Geometry check sheet. Reference: drawing and pictorial views, mm from the part's lowest x, y, z. A direction names the side the tool comes from. Give positions to 0.01 mm unless a question says otherwise; leave off trailing zeros. Write each loop counter-clockwise with the first axis right and the second up, starting at its lowest first coordinate (ties: lowest second). Pieces come first, ordered by that corner, then holes.
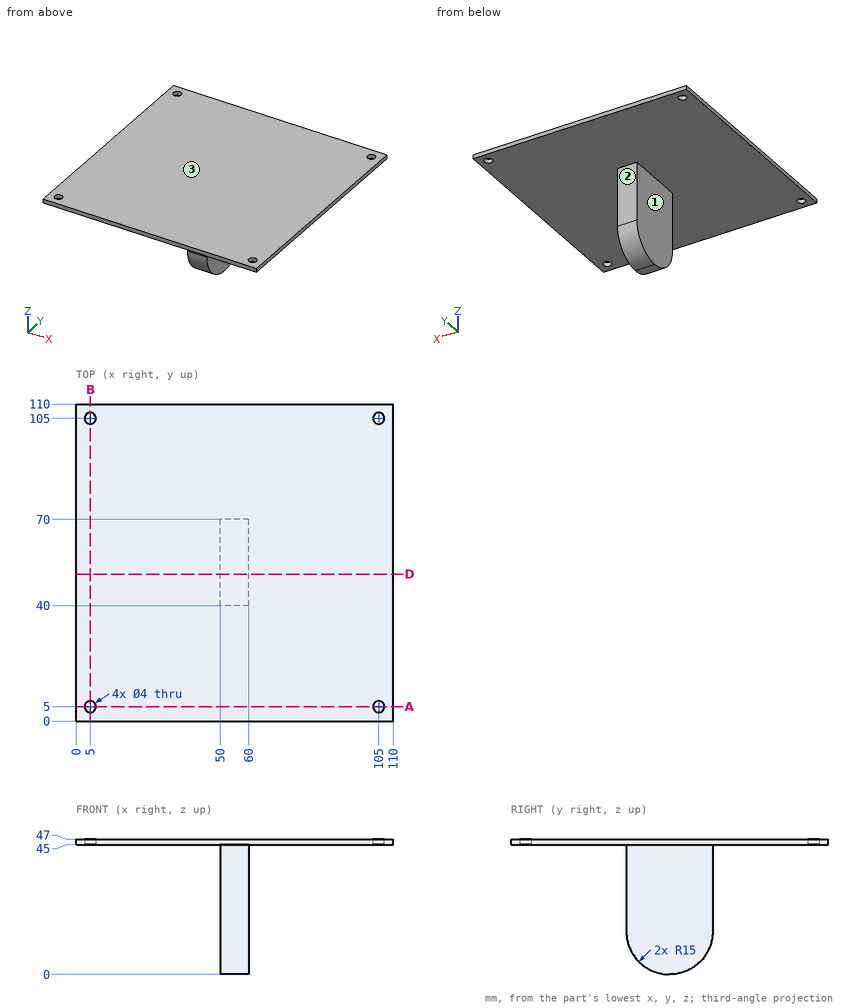
Item 1: Scan lines: line 1 along X through (y, z) = (105, 46); line 2 along Z through (x, y) = (20.5, 54.5). Record each from-to range of solid material in increasing order.
Answer key:
line 1: x = 0 to 3, 7 to 103, 107 to 110
line 2: z = 45 to 47
Item 2: Sectioned sample at D-D on y = 51. Record the cut outline in (x, z).
Answer key:
outline: (0, 45) - (50, 45) - (50, 0.54) - (60, 0.54) - (60, 45) - (110, 45) - (110, 47) - (0, 47) - close
Item 3: Depth check by flat-ended pin: pin 1 (3 mm diameter, centred on x = 13, y = 46, fed in from -Z); pin 2 (11 mm diameter, centred on x = 53, z = 31.5, fed in from +Y); pin 3 (11 mm diameter, centred on x = 52.5, z = 33, fed in from -Y). Enter the tip coordinate at first touch or a pass-through.
Answer key:
pin 1: stops at z = 45
pin 2: stops at y = 70
pin 3: stops at y = 40
Item 4: Set-up check for the marked faces 1, 2 and 3: record each of +Z, -Z, +X, -X, +Y, -Y from which the full face is reachable in a straight line by a thin tool's end or side.
Answer key:
face 1: -Z, -X, +Y, -Y
face 2: -Z, +X, -X, +Y
face 3: +Z, +X, -X, +Y, -Y
Item 5: Sectioned sample at A-A on y = 5. Record the cut outline in (x, z), then the cut area to 3 significant figures.
Answer key:
outline: (0, 45) - (3, 45) - (3, 47) - (0, 47) - close; (7, 45) - (103, 45) - (103, 47) - (7, 47) - close; (107, 45) - (110, 45) - (110, 47) - (107, 47) - close
area: 204 mm2
